Autodesk Inventor part; units mm, degrees
ref_plane "YZ Plane" through (0, 0, 0) normal (1, 0, 0) x (0, 1, 0)
ref_plane "XZ Plane" through (0, 0, 0) normal (0, 1, 0) x (-1, 0, 0)
ref_plane "XY Plane" through (0, 0, 0) normal (0, 0, 1) x (1, 0, 0)
sketch "스케치1" plane through (0, 0, 0) normal (0, 0, 1) x (1, 0, 0)
  line L0 (-3, 0) -> (-1.5, 2.5981)
  line L1 (-1.5, 2.5981) -> (1.5, 2.5981)
  line L2 (1.5, 2.5981) -> (3, 0)
  line L3 (3, 0) -> (1.5, -2.5981)
  line L4 (1.5, -2.5981) -> (-1.5, -2.5981)
  line L5 (-1.5, -2.5981) -> (-3, 0)
  point P0 (0, 0)
  point P1 (0, 0)
  dimension "d0" = 6
extrude "돌출1" add sketch "스케치1" along normal blind 30
sketch "스케치2" plane through (0, 0, 30) normal (0, 0, 1) x (1, 0, 0)
  circle A0 centre (0, 0) radius 1.5
  dimension "d3" = 3
extrude "돌출2" add sketch "스케치2" along normal blind 5
sketch "스케치3" plane through (0, 0, 0) normal (0, 0, -1) x (-1, 0, 0)
  circle A0 centre (0, 0) radius 1.5
  dimension "d6" = 3
extrude "돌출3" cut sketch "스케치3" against normal blind 5
properties part number "50mm지지대"
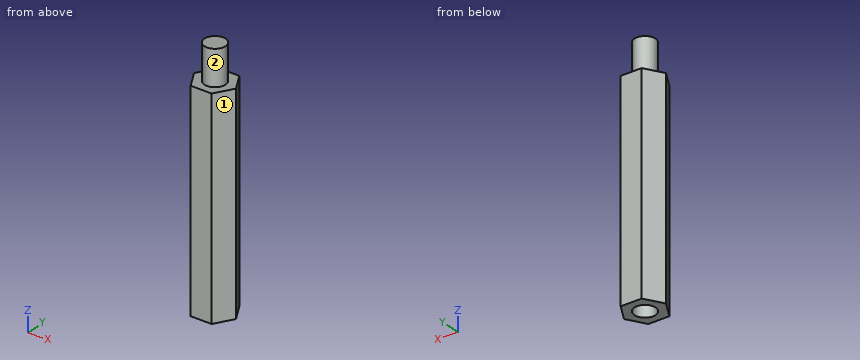
Design review of the part built by this model. Coordinates are the model's own, in mm. Face numbers are marked on the shaded views. A direction names the side the tool comes from. Give positions to 0.01 mm unless a question says otherwise; leave off trailing zeros. Order: outer loops, then holes, each group sorted by start corner. A loop starts at its lowest first (then second) coordinate and runs counter-clockwise, first axis right, second up. Notation, with made-up numbers: (27, -32.5) -> (53, -32.5) arc R29 cw to (53, 3.5) -> close; hole circle Ø5 at (27, -4). An arc over 180 degrees is marked (long way). Write each question's results on one line, items separated by ' | '. Start each with the question number.
Q1. For pin 1 (1.5 mm diameter, centred on y = -1, z = 23.5, fed in from -X); pin 2 (0.9 mm diameter, centred on x = -0.5, y = -0.5, fed in from -Z), all flat-tipped, find the tip position at first contact; note any pin that passes through.
Q2. Add section B-B on y = -0.85. Give the boundary of the cut face in (x, z), and give its area (3 significant figures).
Q3. Add section A-A on x = 0. Give the boundary of the cut face in (y, z).
Q4. Machinability: for the marked faces 1 and 2, which of the approach directions +Z, -Z, +X, -X, +Y, -Y give a long, thin tool a straight path to every point of the face, cutting with its end or side? Answer none if there is none.
Q5. Wall thickness on L1, parallel to Y at x = 0, z = 2.7; L2, parallel to Z at x = -0.65, y = -1.75; L3, parallel to Z at x = 0.6, y = -0.8: over which ranges is each line inside the solid? List them lowest first. Write a range as from..to.
Q6. Add section C-C on z = 14. Give the boundary of the cut face in (x, y).
Found:
1) pin 1: stops at x = -2.86 | pin 2: stops at z = 5
2) outline: (-2.51, 0) -> (-1.24, 0) -> (-1.24, 5) -> (1.24, 5) -> (1.24, 0) -> (2.51, 0) -> (2.51, 30) -> (1.24, 30) -> (1.24, 35) -> (-1.24, 35) -> (-1.24, 30) -> (-2.51, 30) -> close | area: 151 mm2
3) outline: (-2.6, 0) -> (-1.5, 0) -> (-1.5, 5) -> (1.5, 5) -> (1.5, 0) -> (2.6, 0) -> (2.6, 30) -> (1.5, 30) -> (1.5, 35) -> (-1.5, 35) -> (-1.5, 30) -> (-2.6, 30) -> close
4) face 1: +Z, -Z, +X, -Y | face 2: +Z
5) L1: y = -2.6..-1.5, 1.5..2.6 | L2: z = 0..30 | L3: z = 5..35
6) outline: (-3, 0) -> (-1.5, -2.6) -> (1.5, -2.6) -> (3, 0) -> (1.5, 2.6) -> (-1.5, 2.6) -> close
